Autodesk Inventor part; units mm, degrees
ref_plane "Work Plane1" through (0, 5.5, 0) normal (0, 1, 0) x (1, 0, 0)
ref_plane "YZ Plane" through (0, 0, 0) normal (1, 0, 0) x (0, 1, 0)
ref_plane "XZ Plane" through (0, 0, 0) normal (0, 1, 0) x (-1, 0, 0)
sketch "Sketch1" plane through (0, 0, 0) normal (0, 1, 0) x (-1, 0, 0)
  line L0 (0, 0) -> (8, 0)
  line L1 (0, 0) -> (0, 3)
  line L2 (0, 3) -> (8, 3)
  arc A0 (11, -3) -> (8, 0) centre (8, -3) ccw
  arc A1 (14, -3) -> (8, 3) centre (8, -3) ccw
  line L3 (11, -3) -> (11, -11)
  line L4 (11, -11) -> (14, -11)
  line L5 (14, -11) -> (14, -3)
  line L6 (0, 0) -> (11, -11)
  dimension "d0" = 3
  dimension "d1" = 3
  dimension "d2" = 8
  dimension "d3" = 3
  dimension "d4" = 8
extrude "Extrusion1" add sketch "Sketch1" along normal blind 8 contours L1 L2 A1 L5 L4 L3 A0 L0
sketch "Sketch2" plane through (0, 0, 0) normal (0, -1, 0) x (1, 0, 0)
  line L0 (0, 0) -> (-8, 0)
  arc A0 (-8, 0) -> (-11, -3) centre (-8, -3) ccw
  line L1 (-11, -3) -> (-11, -11)
  line L2 (0, 0) -> (-11, -11)
  line L3 (-11, -11) -> (-11, -3)
  line L4 (-8, 0) -> (0, 0)
  arc A1 (-8, 0) -> (-11, -3) centre (-8, -3) ccw
  line L5 (0, 0) -> (0, -8)
  arc A2 (-3, -11) -> (0, -8) centre (-3, -8) ccw
  line L6 (-3, -11) -> (-11, -11)
extrude "Extrusion2" add sketch "Sketch2" against normal blind 2.5
ref_plane "Work Plane1" through (0, 5.5, 0) normal (0, 1, 0) x (1, 0, 0)
sketch "Sketch3" plane through (0, 5.5, 0) normal (0, 1, 0) x (1, 0, 0)
  line L0 (0, 0) -> (0, 8)
  arc A0 (0, 8) -> (-3, 11) centre (-3, 8) ccw
  line L1 (-3, 11) -> (-11, 11)
  line L2 (-11, 3) -> (-11, 11)
  arc A1 (-11, 3) -> (-8, 0) centre (-8, 3) ccw
  line L3 (0, 0) -> (-8, 0)
extrude "Extrusion3" add sketch "Sketch3" along normal blind 2.5
sketch "Sketch4" plane through (0, 8, 0) normal (0, 1, 0) x (1, 0, 0)
  arc A0 (0, 8) -> (-3, 11) centre (-3, 8) ccw
  line L0 (0, -3) -> (0, 8)
  line L1 (-3, 11) -> (-14, 11)
  line L2 (-14, 11) -> (-14, 3)
  arc A1 (-14, 3) -> (-8, -3) centre (-8, 3) ccw
  line L3 (-8, -3) -> (0, -3)
  point P0 (0, 0)
sketch "Sketch5" plane through (0, 8, 0) normal (0, 1, 0) x (1, 0, 0)
  circle A0 centre (-9, 2) radius 1.6667
  line L0 (-8, -3) -> (0, -3)
  line L1 (-14, 11) -> (-14, 3)
  point P0 (0, 0)
  dimension "d21" = 3.3333
  dimension "d22" = 3.3333
  dimension "d23" = 3.3333
extrude "Extrusion4" cut sketch "Sketch5" against normal through all
fillet "Fillet2" radius 0.25 1 edges at (-10.6667, 8, -2)
equation "\"d23\" = d22"
properties part number "Plate Adapter 4.0"
Could you check a few things on this model? Use its own coordinates, in mm. A direction names the side the tool comes from. Coordinates: 2 decimals unless noted, no trailing zeros. Order: outer loops, then holes, each group sorted by start corner. A loop starts at its lowest first (then second) coordinate and runs counter-clockwise, first axis right, second up. Notation, with made-up numbers: (-28.5, 15.5) - (-12.5, 15.5) arc R17 ccw to (-12.5, 46.5) - close; hole circle Ø5 at (-26, 65.25). An arc over 180 degrees is marked (long way). Answer in a Markdown table with one row per item. Add a question column.
(1) If we section it at D-D, the plane y = 4.5: Please give me the cut outline in (x, z).
(2) If we mould it in two halves opening along X, with no side actions, what happens to faces 1 (the face through (-14, 4, -7)), 2 (the face through (-10.323, 3.929, -0.986)), 3 (the face through (-7, 8, -4)), 4 (the face through (-10.89, 3.98, -2.2))? For each: released by +X, released by -X, zero draft, split by the parting line, or undercut.
(3) If we section it at A-A, the plane y = 6.5: Please give me the cut outline in (x, z).
(4) I need wall thicknesses on L1, parallel to Y at x = -5.75, z = -6.75; L2, parallel to X at y = 7.25, z = -1; L3, parallel to X at y = 3.5, z = -6.75. Which ranges of each line are inside material? Lowest first, please.
(5) Will this pin go through, and if not, where does the flat tip stop? pin 1 (0.9 mm diameter, centred on x = -5.5, y = 3.5, fed in from -Z).
(6) If we section it at C-C, the plane x = -9: Please give me the cut outline in (y, z).
(7) On a 3-axis mill with a long thin cutter (end or side, diameter ignored), from which of +Z, -Z, +X, -X, +Y, -Y can I reach the whole of each face in a straight line? I mean faces 5 (the face through (-11, 4, -7)), 6 (the face through (-0.9, 1.23, -10.14)). Say none if no direction works.
(8) If we section it at B-B, the plane z = -2: Please give me the cut outline in (x, y).
Results are:
| question | item | result |
|---|---|---|
| 1 | outline | (-14, -11) - (-11, -11) - (-11, -3) arc R3 cw to (-10.58, -1.47) arc R1.67 cw to (-9.53, -0.42) arc R3 cw to (-8, 0) - (0, 0) - (0, 3) - (-8, 3) arc R6 ccw to (-14, -3) - close |
| 2 | face 1 | released by -X |
| 2 | face 2 | undercut |
| 2 | face 3 | zero draft |
| 2 | face 4 | released by +X |
| 3 | outline | (-14, -11) - (-3, -11) arc R3 ccw to (0, -8) - (0, 3) - (-8, 3) arc R6 ccw to (-14, -3) - close; hole circle Ø3.33 at (-9, -2) |
| 4 | L1 | y = 0 to 2.5, 5.5 to 8 |
| 4 | L2 | x = -13.66 to -10.33, -7.67 to 0 |
| 4 | L3 | x = -14 to -11 |
| 5 | pin 1 | stops at z = 0 |
| 6 | outline | (0, -11) - (2.5, -11) - (2.5, -3.67) - (0, -3.67) - close; (0, -0.33) - (2.5, -0.33) - (2.5, -0.17) - (5.5, -0.17) - (5.5, -0.33) - (7.75, -0.33) arc R0.25 ccw to (8, -0.08) - (8, 2.92) - (0, 2.92) - close; (5.5, -11) - (8, -11) - (8, -3.92) arc R0.25 ccw to (7.75, -3.67) - (5.5, -3.67) - close |
| 7 | face 5 | -Z, +X |
| 7 | face 6 | -Z, +X, +Y, -Y |
| 8 | outline | (-13.92, 0) - (-10.67, 0) - (-10.67, 2.5) - (-10.83, 2.5) - (-10.83, 5.5) - (-10.67, 5.5) - (-10.67, 7.75) arc R0.25 ccw to (-10.92, 8) - (-13.92, 8) - close; (-7.33, 0) - (0, 0) - (0, 2.5) - (-7.33, 2.5) - close; (-7.33, 5.5) - (0, 5.5) - (0, 8) - (-7.08, 8) arc R0.25 ccw to (-7.33, 7.75) - close |
